Work out the finished part from the listing and answer in its coordinate system (mm). Coordinates: 2 decimals unless noted, no trailing zeros. Order: outer loops, then holes, each group sorted by start corner. A loop starts at its lowest first (then second) coordinate and runs counter-clockwise, first axis right, second up. Notation, with made-up numbers: (56.25, 45.25) -> (87.25, 45.25) arc R18 ccw to (87.25, 56.25) -> close; hole circle Ø7 at (-17, 26.25). An arc over 180 degrees is marked (long way). Write item = value, one per line. Start each with the question number.
Q1. Straight lines are drawn through the part: L1, parallel to X at y = -1.45, z = -71; L2, parallel to Z at x = 4.5, y = -3; L3, parallel to Z at x = 42.5, y = -5.25. For each, find the intervals that lie inside material, in ascending order. Write a range as from..to.
Q2. A flat-ended cylindrical pin translates along its axis: pin 1 (2 mm diameter, centred on x = 21.5, z = -21.5, fed in from +Y). Find the tip coordinate at first contact, or state that the pin passes through.
Q3. For a pull along Z with two mould halves and no side action, classify faces 1 (the cylindrical face through (48.5, -3.04, -86.07)), 2 (the cylindrical face through (-48.57, -3.04, 86)), 3 (the flat face through (-1, 0, 1)), 4 (the cylindrical face through (-45.548, -2.958, -80.388)) as +Z half, -Z half, draft (parallel to the pull), parting line (faces both ways), or undercut.
Q4. The part is cut by section A-A, the plane x = -43. Determine the outline of the cut face in (y, z).
```python
from build123d import *

# Parameters (mm, degrees)
F0_W     = 100
F0_H     = 175
F0_R     = 2.55
F1_DEPTH = 6
F2_R     = 5
F3_R     = 0.5
F4_DEPTH = 25


with BuildPart() as f1:
    # F0 (on Front) → F1 (new body)
    with BuildSketch(Plane.XZ):
        Rectangle(F0_W, F0_H)
        with Locations((-43, -80.5)):
            Circle(F0_R, mode=Mode.SUBTRACT)
        with Locations((43, -80.5)):
            Circle(F0_R, mode=Mode.SUBTRACT)
        with Locations((-43, 80.5)):
            Circle(F0_R, mode=Mode.SUBTRACT)
        with Locations((43, 80.5)):
            Circle(F0_R, mode=Mode.SUBTRACT)
    extrude(amount=F1_DEPTH)

    # F2
    f2_edges = [f1.edges().sort_by_distance(p)[0] for p in [
        (-50, -3, 87.5),
        (-50, -3, -87.5),
        (50, -3, 87.5),
        (50, -3, -87.5),
    ]]
    fillet(f2_edges, radius=F2_R)

    # F3 (on face) → F4 (cut)
    with BuildSketch(Plane.XZ.offset(6)):
        with Locations((0, -67)):
            Circle(F3_R)
        with Locations((0, -65)):
            Circle(F3_R)
        with Locations((0, -63)):
            Circle(F3_R)
        with Locations((0, -61)):
            Circle(F3_R)
        with Locations((0, -59)):
            Circle(F3_R)
        with Locations((-1.902113, -66.381966)):
            Circle(F3_R)
        with Locations((-1.175571, -68.618034)):
            Circle(F3_R)
        with Locations((1.175571, -68.618034)):
            Circle(F3_R)
        with Locations((1.902113, -66.381966)):
            Circle(F3_R)
        with Locations((-2.162563, -63.634986)):
            Circle(F3_R)
        with Locations((-3.243845, -61.952479)):
            Circle(F3_R)
        with Locations((-4.325127, -60.269972)):
            Circle(F3_R)
        with Locations((-3.638528, -65.33834)):
            Circle(F3_R)
        with Locations((-5.457792, -64.50751)):
            Circle(F3_R)
        with Locations((-7.277056, -63.67668)):
            Circle(F3_R)
        with Locations((-3.959286, -67.569259)):
            Circle(F3_R)
        with Locations((-5.938929, -67.853889)):
            Circle(F3_R)
        with Locations((-7.918572, -68.138519)):
            Circle(F3_R)
        with Locations((-3.022998, -69.619443)):
            Circle(F3_R)
        with Locations((-4.534497, -70.929164)):
            Circle(F3_R)
        with Locations((-6.045997, -72.238886)):
            Circle(F3_R)
        with Locations((-1.12693, -70.837972)):
            Circle(F3_R)
        with Locations((-1.690395, -72.756958)):
            Circle(F3_R)
        with Locations((-2.25386, -74.675944)):
            Circle(F3_R)
        with Locations((1.12693, -70.837972)):
            Circle(F3_R)
        with Locations((1.690395, -72.756958)):
            Circle(F3_R)
        with Locations((2.25386, -74.675944)):
            Circle(F3_R)
        with Locations((3.022998, -69.619443)):
            Circle(F3_R)
        with Locations((4.534497, -70.929164)):
            Circle(F3_R)
        with Locations((6.045997, -72.238886)):
            Circle(F3_R)
        with Locations((3.959286, -67.569259)):
            Circle(F3_R)
        with Locations((5.938929, -67.853889)):
            Circle(F3_R)
        with Locations((7.918572, -68.138519)):
            Circle(F3_R)
        with Locations((3.638528, -65.33834)):
            Circle(F3_R)
        with Locations((5.457792, -64.50751)):
            Circle(F3_R)
        with Locations((7.277056, -63.67668)):
            Circle(F3_R)
        with Locations((2.162563, -63.634986)):
            Circle(F3_R)
        with Locations((3.243845, -61.952479)):
            Circle(F3_R)
        with Locations((4.325127, -60.269972)):
            Circle(F3_R)
    extrude(amount=-F4_DEPTH, mode=Mode.SUBTRACT)


solid = f1.part
```
Model answer:
q1.L1 = -50..-5.03, -4.04..-1.6, -0.65..0.65, 1.6..4.04, 5.03..50
q1.L2 = -87.5..-71.43, -70.43..-60.74, -59.8..87.5
q1.L3 = -87.5..-83, -78..78, 83..87.5
q2.pin_1 = 0
q3.face_1 = -Z half
q3.face_2 = +Z half
q3.face_3 = draft
q3.face_4 = undercut
q4.outline = (-6, -87.5) -> (0, -87.5) -> (0, -83.05) -> (-6, -83.05) -> close; (-6, -77.95) -> (0, -77.95) -> (0, 77.95) -> (-6, 77.95) -> close; (-6, 83.05) -> (0, 83.05) -> (0, 87.5) -> (-6, 87.5) -> close
